The listing builds one solid part. Answer for the finished solid, in the listing's coordinates (mm). Face numbers are marked on the shaded views. A direction names the side the tool comes from. Round coordinates to 2 decimals unless told otherwise and drop trailing zeros. Loops run counter-clockwise (first coordinate to the right, second up) from the corner with the lowest first, then second, coordinate; pieces in that order, holes last. Notation, with made-up numbers: (22, -30) -> (76, -30) arc R21 ccw to (76, -12) -> close; hole circle Ø8 at (89, 38). An arc over 180 degrees is marked (long way). Use a Markdown table: item, result. Add a question column.
Q1. For a pull along X with two mould halves and no side action, classify the marked faces 3, 4 and 5 as released by +X, released by -X, zero draft, split by the parting line, or undercut.
Q2. Given pin 1 Ø2 at (y, z) = (4, 3) entering from +X; pin 2 Ø1.5 at (x, y) = (-2.5, 2) entering from +Z, each flat-ended and moving along its own axis, determine where each tip first touches the part or whether it passes through.
Q3. Consider line 1 (X direction, y = 1.8, z = 0) (3 decimals); line 2 (X direction, y = 4.4, z = -0.5); line 3 (X direction, y = 2.4, z = 5). Determine where each line is inside the solid, lowest interval first.
Q4. Section A-A on z = 0 is taken. Give the vertices of the cut face in (x, y) (3 decimals), then the cut area to 4 significant figures.
Q5. Which of the six approach directions +Z, -Z, +X, -X, +Y, -Y give full straight-line access (tool end or side, diameter ignored) to the marked faces 1 and 2?
Q6. Section B-B on y = 2.75 is taken. Give the number of separate pieces and of enclosed holes in the cut face, then the cut area to 3 significant figures.
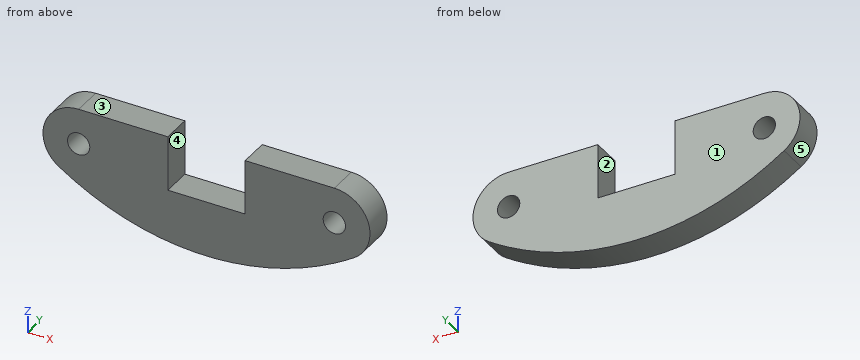
from build123d import *

# Parameters (mm, degrees)
SKETCH1_R           = 1.875
BOSS_EXTRUDE1_DEPTH = 5


with BuildPart() as part:
    # Sketch1 → Boss-Extrude1 (new body)
    with BuildSketch(Plane(origin=(0, 0, 0), x_dir=(1, 0, 0), z_dir=(0, 1, 0))):
        with BuildLine():
            Line((21.5, -6), (6.5, -6))
            Line((6.5, -6), (6.5, -3.25))
            Line((6.5, -3.25), (6.5, 3.25))
            Line((6.5, 3.25), (-6.5, 3.25))
            Line((-6.5, 3.25), (-6.5, -3.25))
            Line((-6.5, -3.25), (-6.5, -6))
            Line((-6.5, -6), (-21.5, -6))
            ThreePointArc((-21.5, -6), (-27.244562647, -1.732050808), (-24.81662479, 5))
            add(Edge.make_bspline(
                [(-24.81662479, 5), (-8.736295123, 15.666484002), (10.378585258, 14.577111967), (24.81662479, 5)],
                knots=[0, 0, 0, 0, 1, 1, 1, 1], degree=3))
            ThreePointArc((24.81662479, 5), (27.244562647, -1.732050808), (21.5, -6))
        make_face()
        with Locations(Location((-21.5, 0, 0), (0, 0, 270))):
            Circle(SKETCH1_R, mode=Mode.SUBTRACT)
        with Locations(Location((21.5, 0, 0), (0, 0, 90))):
            Circle(SKETCH1_R, mode=Mode.SUBTRACT)
    extrude(amount=BOSS_EXTRUDE1_DEPTH)


solid = part.part
Checked values:
| question | item | result |
|---|---|---|
| 1 | face 3 | zero draft |
| 1 | face 4 | undercut |
| 1 | face 5 | released by -X |
| 2 | pin 1 | stops at x = 27.16 |
| 2 | pin 2 | stops at z = -3.25 |
| 3 | line 1 | x = -27.5 to -23.375, -19.625 to -6.5, 6.5 to 19.625, 23.375 to 27.5 |
| 3 | line 2 | x = -27.48 to -23.31, -19.69 to -6.5, 6.5 to 19.69, 23.31 to 27.48 |
| 3 | line 3 | x = -24.82 to -6.5, 6.5 to 24.82 |
| 4 | outline | (-27.5, 0) -> (-23.375, 0) -> (-23.375, 5) -> (-27.5, 5) -> close; (-19.625, 0) -> (-6.5, 0) -> (-6.5, 5) -> (-19.625, 5) -> close; (6.5, 0) -> (19.625, 0) -> (19.625, 5) -> (6.5, 5) -> close; (23.375, 0) -> (27.5, 0) -> (27.5, 5) -> (23.375, 5) -> close |
| 4 | area | 172.5 mm2 |
| 5 | face 1 | +Z, -Z, +X, -X, +Y |
| 5 | face 2 | +Z, +Y, -Y |
| 6 | separate pieces | 1 |
| 6 | enclosed holes | 2 |
| 6 | area | 694 mm2 |
